Autodesk Inventor part; units mm, degrees
ref_plane "YZ Plane" through (0, 0, 0) normal (1, 0, 0) x (0, 1, 0)
ref_plane "XZ Plane" through (0, 0, 0) normal (0, 1, 0) x (-1, 0, 0)
ref_plane "XY Plane" through (0, 0, 0) normal (0, 0, 1) x (1, 0, 0)
sketch "Sketch1" plane through (0, 0, 0) normal (0, 1, 0) x (-1, 0, 0)
  circle A0 centre (0, 0) radius 1.5
  line L0 (0, 0) -> (0, -15)
  line L1 (0, 0) -> (15, 0) construction
  circle A1 centre (0, -15) radius 1.5
  line L2 (0, -15) -> (0, -17.5)
  line L3 (0, -17.5) -> (0, -20)
  circle A2 centre (0, 0) radius 3
  line L4 (3, 0) -> (-3, 0)
  line L5 (-3, 0) -> (-3, -20)
  line L6 (-3, -20) -> (3, -20)
  line L7 (3, -20) -> (3, 0)
  dimension "d6" = 6
  dimension "d0" = 3
  dimension "d1" = 15
  dimension "d2" = 90
  dimension "d3" = 3
  dimension "d4" = 2.5
  dimension "d5" = 2.5
sketch "Sketch1 outline for Extrusion1" plane through (0, 0, 0) normal (0, 1, 0) x (-1, 0, 0)
  arc A0 (3, 0) -> (-3, 0) centre (0, 0) ccw
  line L0 (3, -20) -> (3, 0)
  line L1 (-3, 0) -> (-3, -20)
  line L2 (-3, -20) -> (3, -20)
  circle A1 centre (0, -15) radius 1.5
  circle A2 centre (0, 0) radius 1.5
extrude "Extrusion1" add sketch "Sketch1 outline for Extrusion1" along normal blind 2.5
sketch "Sketch2" plane through (0, 2.5, 0) normal (0, 1, 0) x (1, 0, 0)
  line L0 (3, 20) -> (-3, 20)
  line L1 (-3, 20) -> (3, 20)
  line L2 (3, 20) -> (3, 17.7)
  line L3 (3, 17.7) -> (-3, 17.7)
  line L4 (-3, 17.7) -> (-3, 20)
  point P0 (0, 0)
  dimension "d9" = 2.3
sketch "Sketch2 outline for Extrusion2" plane through (0, 2.5, 0) normal (0, 1, 0) x (1, 0, 0)
  line L0 (-3, 20) -> (-3, 17.7)
  line L1 (3, 20) -> (-3, 20)
  line L2 (3, 17.7) -> (3, 20)
  line L3 (-3, 17.7) -> (3, 17.7)
extrude "Extrusion2" add sketch "Sketch2 outline for Extrusion2" along normal blind 10
sketch "Sketch3" plane through (3, 0, -20) normal (0, 0, -1) x (-1, 0, 0)
  line L0 (0, 0) -> (0, 12.5)
  line L1 (6, 0) -> (6, 12.5)
  line L2 (0, 12.5) -> (6, 12.5)
  line L3 (6, 12.5) -> (6, 10.5)
  line L4 (6, 10.5) -> (0, 10.5)
  line L5 (0, 10.5) -> (0, 12.5)
  line L6 (0, 10.5) -> (6, 10.5)
  line L7 (6, 10.5) -> (6, 6.5)
  line L8 (6, 6.5) -> (0, 6.5)
  line L9 (0, 6.5) -> (0, 10.5)
  line L10 (0, 6.5) -> (6, 6.5)
  line L11 (6, 6.5) -> (6, 4.5)
  line L12 (6, 4.5) -> (0, 4.5)
  line L13 (0, 4.5) -> (0, 6.5)
  point P0 (3, 0)
  point P1 (0, 4.5)
  point P2 (0, 6.5)
  point P3 (0, 10.5)
  dimension "d12" = 2
  dimension "d13" = 6
  dimension "d14" = 4
  dimension "d15" = 2
sketch "Sketch3 outline for Extrusion3" plane through (3, 0, -20) normal (0, 0, -1) x (-1, 0, 0)
  line L0 (0, 4.5) -> (6, 4.5)
  line L1 (0, 6.5) -> (0, 4.5)
  line L2 (6, 6.5) -> (0, 6.5)
  line L3 (6, 4.5) -> (6, 6.5)
  line L4 (6, 12.5) -> (0, 12.5)
  line L5 (6, 10.5) -> (6, 12.5)
  line L6 (0, 10.5) -> (6, 10.5)
  line L7 (0, 12.5) -> (0, 10.5)
extrude "Extrusion3" add sketch "Sketch3 outline for Extrusion3" along normal blind 3
sketch "Sketch4" plane through (3, 0, 0) normal (1, 0, 0) x (0, 0, -1)
  line L0 (20, 10.5) -> (23, 10.5)
  line L1 (20, 6.5) -> (23, 6.5)
  line L2 (23, 10.5) -> (22.5, 10.5)
  line L3 (22.5, 10.5) -> (22.5, 6.5)
  line L4 (22.5, 6.5) -> (23, 6.5)
  line L5 (23, 6.5) -> (23, 10.5)
  line L6 (22.5, 10.5) -> (23.5, 10.5)
  line L7 (23.5, 10.5) -> (23.5, 9.5)
  line L8 (23.5, 9.5) -> (22.5, 9.5)
  line L9 (22.5, 9.5) -> (22.5, 10.5)
  line L10 (22.5, 6.5) -> (23.5, 6.5)
  line L11 (23.5, 6.5) -> (23.5, 7.5)
  line L12 (23.5, 7.5) -> (22.5, 7.5)
  line L13 (22.5, 7.5) -> (22.5, 6.5)
  line L14 (23, 12.5) -> (23, 10.5)
  line L15 (23.5, 10.5) -> (23, 12.5)
  line L16 (23, 12.5) -> (23, 10.5)
  line L17 (23.5, 6.5) -> (23, 4.499196)
  line L18 (23, 4.5) -> (23, 6.5)
  line L19 (23, 4.499196) -> (23, 6.5)
  point P0 (0, 0)
  dimension "d18" = 0.5
  dimension "d19" = 1
  dimension "d20" = 1
  dimension "d21" = 1
  dimension "d22" = 1
sketch "Sketch4 outline for Extrusion4" plane through (3, 0, 0) normal (1, 0, 0) x (0, 0, -1)
  line L0 (23, 4.5) -> (23.5, 6.5)
  line L1 (23, 6.5) -> (23, 4.5)
  line L2 (22.5, 6.5) -> (23, 6.5)
  line L3 (22.5, 7.5) -> (22.5, 6.5)
  line L4 (23.5, 7.5) -> (22.5, 7.5)
  line L5 (23.5, 6.5) -> (23.5, 7.5)
  line L6 (22.5, 9.5) -> (23.5, 9.5)
  line L7 (22.5, 10.5) -> (22.5, 9.5)
  line L8 (23, 10.5) -> (22.5, 10.5)
  line L9 (23, 12.5) -> (23, 10.5)
  line L10 (23.5, 10.5) -> (23, 12.5)
  line L11 (23.5, 9.5) -> (23.5, 10.5)
extrude "Extrusion4" add sketch "Sketch4 outline for Extrusion4" against normal blind 6
fillet "Fillet1" radius 2 5 edges at (0, 12.5, -23) (0, 12.5, -17.7) (0, 4.5, -23) (0, 4.5, -20) (0, 0, -20)
properties part number "wire_holder_femur"
Read the model definition and answer for the solid it produces. Units are mm, in the model's axes. A direction names the side the tool comes from. Round coordinates to 2 decimals unless told otherwise and drop trailing zeros. Loops run counter-clockwise (first coordinate to the right, second up) from the corner with the lowest first, then second, coordinate; pieces in that order, holes last.
Q1. Which of the six approach directions +Z, -Z, +X, -X, +Y, -Y give full straight-line access (tool end or side, diameter ignored) to faces 5 (the face through (0, 9.5, -23)), 6 (the face through (0, 10.5, -21)), 7 (the face through (0, 0, -7))?
Q2. Section A-A on z = -15 is taken. Write down the section's boundary in (x, y).
Q3. Section C-C on y = 1.5 is taken. Write down the section's boundary in (x, z).
Q4. Each of these flat-tipped pins is pushed along its axis until it touches: pin 1 (0.5 mm diameter, centred on x = 1, y = 10, fed in from +Z); pin 2 (2.5 mm diameter, centred on x = 0, z = 0, fed in from -Y); pin 3 (0.5 mm diameter, centred on x = -1, z = -23, fed in from +Y); pin 4 (1.2 mm diameter, centred on x = -0.5, z = -21, fed in from -Y). Where does it stop, or does it pass through?
Q5. Section D-D on z = 0.75 is taken. Write down the section's boundary in (x, y), and give its area (3 significant figures).
Q6. Consider probe 1 along Z at (x, y) = (0, 0.85); probe 2 along Z at (x, y) = (0, 1.6); probe 3 along Y at (x, z) = (-2.25, -5.5). Determine where each line is inside the solid, lowest interval first.
Q7. Section B-B on x = 0 is taken. Give the number of separate pieces and of enclosed holes in the cut face, and give its area (3 significant figures).
Q8. Determine the mould class of faces 1 (the face through (0, 7, -22.5)), 2 (the face through (0, 10, -22.5)), 3 (the face through (0, 2.5, -7)), 4 (the face through (-0.042, 3.794, -20.475)) for opening direction Y: released by +Y, released by -Y, zero draft, split by the parting line, or undercut.
Output:
1. face 5: -Z, +X, -X
1. face 6: +X, -X
1. face 7: +Z, -Z, +X, -X, -Y
2. outline: (-3, 0) - (-1.5, 0) - (-1.5, 2.5) - (-3, 2.5) - close; (1.5, 0) - (3, 0) - (3, 2.5) - (1.5, 2.5) - close
3. outline: (-3, -19.94) - (3, -19.94) - (3, 0) arc R3 ccw to (-3, 0) - close; hole circle Ø3 at (0, -15); hole circle Ø3 at (0, 0)
4. pin 1: stops at z = -17.7
4. pin 2: passes through
4. pin 3: stops at y = 12.01
4. pin 4: stops at y = 3.7
5. outline: (-2.9, 0) - (-1.3, 0) - (-1.3, 2.5) - (-2.9, 2.5) - close; (1.3, 0) - (2.9, 0) - (2.9, 2.5) - (1.3, 2.5) - close
5. area: 8.03 mm2
6. probe 1: z = -19.64 to -16.5, -13.5 to -1.5, 1.5 to 3
6. probe 2: z = -19.96 to -16.5, -13.5 to -1.5, 1.5 to 3
6. probe 3: y = 0 to 2.5
7. separate pieces: 3
7. enclosed holes: 0
7. area: 78.8 mm2
8. face 1: undercut
8. face 2: undercut
8. face 3: released by +Y
8. face 4: released by -Y
